from build123d import *

# Parameters (mm, degrees)
ESQUISSE1_W             = 2.25
ESQUISSE1_H             = 40
ENL_V_MAT_EXTRU_1_DEPTH = 3


with BuildPart() as part:
    # Esquisse1 → Révolution1 (revolve)
    with BuildSketch(Plane.XY, mode=Mode.PRIVATE) as r_volution1_sk:
        Rectangle(ESQUISSE1_W, ESQUISSE1_H)
        Polygon((-2.875, 20), (-1.125, 20), (1.125, 20), (1.125, 24), (-2.875, 24), align=None)
    revolve(r_volution1_sk.sketch.rotate(Axis((1.125, -20, 0), (0, 1, 0)), 270), axis=Axis((1.125, -20, 0), (0, 1, 0)))

    # Esquisse2 → Enlèv. mat.-Extru.1 (cut)
    with BuildSketch(Plane(origin=(0, 24, 0), x_dir=(1, 0, 0), z_dir=(0, 1, 0))):
        Polygon((3.434401077, 0), (2.279700538, 2), (-0.029700538, 2), (-1.184401077, 0), (-0.029700538, -2), (2.279700538, -2), align=None)
    extrude(amount=-ENL_V_MAT_EXTRU_1_DEPTH, mode=Mode.SUBTRACT)


solid = part.part
Verification items for the finished model (mm, model axes). A direction names the side the tool comes from. Coordinates: 2 decimals unless noted, no trailing zeros. Loops run counter-clockwise (first coordinate to the right, second up) from the corner with the lowest first, then second, coordinate; pieces in that order, holes last. Notation, with made-up numbers: (-19.75, 2) -> (38.25, 2) arc R8 ccw to (38.25, 16) -> close; hole circle Ø9 at (53, 39). An arc over 180 degrees is marked (long way). Answer as a JSON object with one key per item and string values. Group by question number.
Item 1: Sectioned sample at C-C on y = 2. Record the boundary of the cut face in (x, z) (3 decimals).
Item 2: Sectioned sample at A-A on z = 1.25. Record the boundary of the cut face in (x, y).
Item 3: Sectioned sample at B-B on x = 3. Record the boundary of the cut face in (y, z), plus the area to 3 significant figures.
Item 4: Depth check by flat-ended pin: pin 1 (3 mm diameter, centred on x = -1, y = 0.5, fed in from -Z); pin 2 (3 mm diameter, centred on y = 18, z = -1, fed in from -X) (3 decimals); pin 3 (1 mm diameter, centred on y = -12.5, z = 2.5, fed in from -X). Enter the tip coordinate at first touch or a pass-through.
Item 5: Sectioned sample at D-D on x = -2. Record the boundary of the cut face in (y, z), plus the area to 3 significant figures.
Item 6: Scan lines: probe 1 along Y at (x, z) = (0.5, 3); probe 2 along Y at (x, z) = (0.5, -0.25); probe 3 along Z at (x, y) = (-0.75, -14). Record each from-to range of solid material in increasing order.
Item 7: Mould release check, pull along X, two halves, no side actions. Record for faces 4 (the flat face through (-1, 24, 1)), 5 (the flat face through (1, 23, -2)), 6 (the cylindrical face through (-2.84, 21.97, 0.52)): +X half, -X half, draft (parallel to the pull), parting line (faces both ways), or undercut.
Item 8: Tool access check on faces 1 (the flat face through (2.865, 22.521, -0.986)), 2 (the flat face through (3, 20, -2)), 3 (the flat face through (1, -20, 0)). Record the directions out of +Z, -Z, +X, -X, +Y, -Y that give a thin tool (end or side, any length) a straight path to the whole face; none if there is none.
Evaluation:
{
 "1": {"outline": "circle Ø4.5 at (1.125, 0)"},
 "2": {"outline": "(-2.67, 20) -> (-0.75, 20) -> (-0.75, -20) -> (3, -20) -> (3, 20) -> (4.92, 20) -> (4.92, 24) -> (2.71, 24) -> (2.71, 21) -> (-0.46, 21) -> (-0.46, 24) -> (-2.67, 24) -> close"},
 "3": {"outline": "(-20, -1.24) -> (20, -1.24) -> (20, -3.53) -> (24, -3.53) -> (24, -0.75) -> (21, -0.75) -> (21, 0.75) -> (24, 0.75) -> (24, 3.53) -> (20, 3.53) -> (20, 1.24) -> (-20, 1.24) -> close", "area": "123 mm²"},
 "4": {"pin 1": "stops at z = -2.16", "pin 2": "stops at x = -1.125", "pin 3": "stops at x = 0.09"},
 "5": {"outline": "(20, -2.5) -> (24, -2.5) -> (24, 2.5) -> (20, 2.5) -> close", "area": "20.0 mm²"},
 "6": {"probe 1": "y = 20 to 24", "probe 2": "y = -20 to 21", "probe 3": "z = -1.24 to 1.24"},
 "7": {"face 4": "draft", "face 5": "undercut", "face 6": "parting line"},
 "8": {"face 1": "+Y", "face 2": "-Y", "face 3": "+Z, -Z, +X, -X, -Y"}
}
